The listing builds one solid part. Answer for the finished solid, in the listing's coordinates (mm). A direction names the side the tool comes from. Round coordinates to 2 decimals unless told otherwise and drop trailing zeros. Loops run counter-clockwise (first coordinate to the right, second up) from the corner with the lowest first, then second, coordinate; pieces in that order, holes last. Notation, with made-up numbers: (20.25, -4.75) -> (43.25, -4.75) arc R11 cw to (43.25, 12.25) -> close; hole circle Ø3 at (72.25, 68). An arc over 180 degrees is marked (long way). Write each question's results on one line, items separated by ' | '. Start each with the question number.
(1) Straight lines are drawn through the part: probe 1 along Y at (x, z) = (-4, 4.25); probe 2 along Z at (x, y) = (-6.25, 3.5). For each, find the intervals that lie inside material, in ascending order.
(2) Flat-ended cylindrical pins translate along their axes: pin 1 (6 mm diameter, centred on y = 4, z = 15, fed in from -X); pin 2 (3 mm diameter, centred on y = 0, z = 14.5, fed in from -X); pin 3 (1.5 mm diameter, centred on x = 0, y = -1, fed in from -Z); pin 4 (4 mm diameter, centred on x = 6, z = 13.5, fed in from -Y). Find the tip coordinate at first contact, or state that the pin passes through.
(3) Determine the mould class of faces 4 (the face through (0, -8, 5)), 5 (the face through (-3, 0, 15)), 6 (the face through (-5, 0, 4)), 7 (the face through (1.18, -0.89, 15.07)) for opening direction X: released by +X, released by -X, zero draft, split by the parting line, or undercut.
(4) The part is cut by section D-D (y = 2.25). Determine the outline of the cut face in (x, z).
(5) The part is cut by section C-C (z = 18). Determine the outline of the cut face in (x, y).
(6) The part is cut by section A-A (x = -4.25). Determine the outline of the cut face in (y, z), plus the area to 3 significant figures.
(7) For faces 1 (the face through (1.24, 0.806, 15.07)), 2 (the face through (5, 0, 4)), 3 (the face through (2, 0, 10)), determine the directions among +Z, -Z, +X, -X, +Y, -Y from which every point of the face is accessible in a straight line to the end or side of a thin tool.
```python
from build123d import *

# Parameters (mm, degrees)
BOX001_W                 = 10
BOX001_H                 = 10
BOX001_DEPTH             = 8
CYLINDER_W               = 3
CYLINDER_H               = 10
CYLINDER_ANGLE           = 290
CYLINDER_PLACEMENT_ANGLE = 33
BOX_W                    = 16
BOX_H                    = 16
BOX_DEPTH                = 10


with BuildPart() as cube001:
    # Box001 → Box001 (new body)
    with BuildSketch(Plane(origin=(-5, -5, 0), x_dir=(1, 0, 0), z_dir=(0, 0, 1))):
        with Locations((5, 5)):
            Rectangle(BOX001_W, BOX001_H)
    extrude(amount=BOX001_DEPTH)


with BuildPart() as cylinder:
    # Cylinder → Cylinder (revolve)
    with BuildSketch(Plane.XZ):
        with Locations((1.5, 5)):
            Rectangle(CYLINDER_W, CYLINDER_H)
    revolve(axis=Axis((0, 0, 0), (0, 0, 1)), revolution_arc=CYLINDER_ANGLE)


with BuildPart() as cylinder_1:
    # Cylinder placement: moved
    add(cylinder.part.moved(Location((0, 0, 10))).rotate(Axis((0, 0, 10), (0, 0, 1)), CYLINDER_PLACEMENT_ANGLE))


with BuildPart() as cut:
    # Box → Box (new body)
    with BuildSketch(Plane(origin=(-8, -8, 0), x_dir=(1, 0, 0), z_dir=(0, 0, 1))):
        with Locations((8, 8)):
            Rectangle(BOX_W, BOX_H)
    extrude(amount=BOX_DEPTH)

    # Fusion: union Cylinder
    add(cylinder_1.part)

    # Cut: cut Cube001
    add(cube001.part, mode=Mode.SUBTRACT)


solid = cut.part
```
Checked values:
1) probe 1: y = -8 to -5, 5 to 8 | probe 2: z = 0 to 10
2) pin 1: stops at x = -2.83 | pin 2: stops at x = -3 | pin 3: stops at z = 8 | pin 4: passes through
3) face 4: zero draft | face 5: split by the parting line | face 6: undercut | face 7: released by +X
4) outline: (-8, 0) -> (-5, 0) -> (-5, 8) -> (5, 8) -> (5, 0) -> (8, 0) -> (8, 10) -> (1.98, 10) -> (1.98, 20) -> (-1.98, 20) -> (-1.98, 10) -> (-8, 10) -> close
5) outline: (0, 0) -> (2.52, 1.63) arc R3 ccw (long way) to (2.4, -1.81) -> close
6) outline: (-8, 0) -> (-5, 0) -> (-5, 8) -> (5, 8) -> (5, 0) -> (8, 0) -> (8, 10) -> (-8, 10) -> close | area: 80.0 mm2
7) face 1: +Z, +X | face 2: -Z | face 3: +Z
